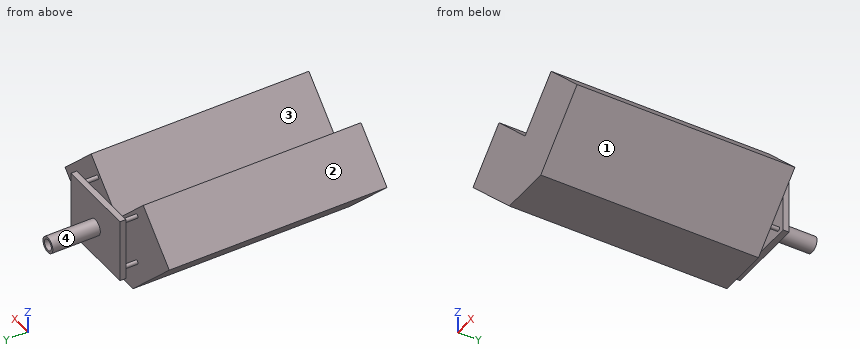
```python
from build123d import *

# Parameters (mm, degrees)
F0_R     = 20
F0_R_2   = 14
F1_DEPTH = 60
F3_W     = 200
F3_H     = 160
F4_DEPTH = 15
F5_R     = 5
F6_DEPTH = 40
F8_DEPTH = 550


with BuildPart() as f1:
    # F0 (on Front) → F1 (new body, symmetric)
    with BuildSketch(Plane.XZ):
        Circle(F0_R)
        Circle(F0_R_2, mode=Mode.SUBTRACT)
    extrude(amount=F1_DEPTH, both=True)

    # F3 (on offset) → F4 (join)
    with BuildSketch(Plane.XZ.offset(60)):
        Rectangle(F3_W, F3_H)
    extrude(amount=F4_DEPTH)

    # F5 (on face) → F6 (join)
    with BuildSketch(Plane.XZ.offset(75)):
        with Locations((-80, 60)):
            Circle(F5_R)
        with Locations((-80, -65)):
            Circle(F5_R)
        with Locations((80, -65)):
            Circle(F5_R)
        with Locations((80, 60)):
            Circle(F5_R)
    extrude(amount=F6_DEPTH)

    # F7 (on face) → F8 (join)
    with BuildSketch(Plane.XZ.offset(115)):
        Polygon((0, 0), (-106.066017, 106.066017), (-212.132034, 0), (-63.983719, -148.148316), (63.983719, -148.148316), (212.132034, 0), (106.066017, 106.066017), align=None)
    extrude(amount=F8_DEPTH)


solid = f1.part
```
Design review of the part built by this model. Coordinates are the model's own, in mm. Face numbers are marked on the shaded views. Give positions to 0.01 mm unless a question says otherwise; leave off trailing zeros. Loops run counter-clockwise (first coordinate to the right, second up) from the corner with the lowest first, then second, coordinate; pieces in that order, holes last. Notation, with made-up numbers: M 55.5,4 L 62.5,4 A12 cw 62.5,12 Z; hole C 40.25,34 d2. An arc over 180 degrees is marked long. Return JSON: item names as keys, results as strings. Group by question number.
Item 1: We need section A-A (x = 54.5). Give the boundary of the cut face in (y, z), and give its area (3 significant figures).
Item 2: For probe 1 along Y at (x, z) = (69, -61); probe 2 along Y at (x, z) = (-17.5, 0.5); probe 3 along Z at (x, y) = (0, -8), list the stretches that pass through material, from the lowest coordinate up.
Item 3: Insertion check: pin 1 Ø12 at (y, z) = (-67.5, -38) entering from +X; pin 2 Ø12 at (y, z) = (-66.5, -26) entering from -X; pin 3 Ø1.5 at (x, z) = (63.5, -67) entering from +Y. Each pin has a flat end and moves straight along its axis. Give the tip position at first contact, or say it passes through.
Item 4: We need section D-D (y = -93). Give the boundary of the cut face in (x, z).
Item 5: We need section B-B (y = -174). Give the boundary of the cut face in (x, z), and give its area (3 significant figures).
Item 6: Mouldability with a two-part tool opening along X and no side actions: class the marked faces 1, 2, 3 and 4 as released by +X, released by -X, zero draft, split by the parting line, or undercut.
Item 7: We need section C-C (z = -41.5). Give the boundary of the cut face in (x, y), and give its area (3 significant figures).
Output:
{
 "1": {"outline": "M -665,-148.15 L -115,-148.15 L -115,54.5 L -665,54.5 Z; M -75,-80 L -60,-80 L -60,80 L -75,80 Z", "area": "114,000 mm^2"},
 "2": {"probe 1": "y = -665 to -115, -75 to -60", "probe 2": "y = -665 to -115, -75 to 60", "probe 3": "z = -20 to -14, 14 to 20"},
 "3": {"pin 1": "stops at x = 100", "pin 2": "stops at x = -100", "pin 3": "stops at y = -60"},
 "4": {"outline": "C -80,-65 d10; C -80,60 d10; C 80,-65 d10; C 80,60 d10"},
 "5": {"outline": "M -212.13,0 L -63.98,-148.15 L 63.98,-148.15 L 212.13,0 L 106.07,106.07 L 0,0 L -106.07,106.07 Z", "area": "63,400 mm^2"},
 "6": {"face 1": "released by +X", "face 2": "released by -X", "face 3": "undercut", "face 4": "split by the parting line"},
 "7": {"outline": "M -170.63,-665 L 170.63,-665 L 170.63,-115 L -170.63,-115 Z; M -100,-75 L 100,-75 L 100,-60 L -100,-60 Z", "area": "191,000 mm^2"}
}
